Part model, mm, in its own coordinate system. A direction names the side the tool comes from. Coordinates: 2 decimals unless noted, no trailing zeros. Loops run counter-clockwise (first coordinate to the right, second up) from the corner with the lowest first, then second, coordinate; pieces in that order, holes last. Notation, with made-up numbers: M -10,58 L 34,58 A26 cw 34,89 Z; hole C 55.25,83 d3. An arc over 180 degrees is marked long. Use a Markdown table: item, result. Add a question column.
1) Band-saw the part on A-A (x = -15.5). List the corners of the cut face in (y, z), plus the area to 3 significant figures.
2) Pull direction Z, two halves, no side cores. Call faces 1 (the flat face through (-10, 1, -1)), 2 (the flat face through (-10, 1, -22)), 3 (the flat face through (-10, 2.5, -11)): released by +Z, released by -Z, zero draft, split by the parting line, or undercut.
3) Tool access for faces 4 (the flat face through (-20, 0.7, -0.5)), 5 (the flat face through (-10, 1, -21)), 6 (the flat face through (0, 0.7, -21.5)): list every direction of +Z, -Z, +X, -X, +Y, -Y with a clear straight run to the whole face (end or side of a thin tool).
4) Wall check: probe 1 along Z at (x, y) = (-13.5, 1.3); probe 2 along Y at (x, z) = (-15.5, -18). Give the ranges that are in metal, low to high. Write a range as from..to.
5) Band-saw the part on B-B (z = -14.75). List the corners of the cut face in (x, y), plus the area to 3 significant figures.
Autodesk Inventor part; units mm, degrees
ref_plane "YZ Plane" through (0, 0, 0) normal (1, 0, 0) x (0, 1, 0)
ref_plane "XZ Plane" through (0, 0, 0) normal (0, 1, 0) x (-1, 0, 0)
ref_plane "XY Plane" through (0, 0, 0) normal (0, 0, 1) x (1, 0, 0)
sketch "Skizze1" plane through (0, 0, 0) normal (0, 1, 0) x (-1, 0, 0)
  point P0 (0, 0)
sketch "Skizze2" plane through (0, 0, 0) normal (0, 1, 0) x (-1, 0, 0)
  line L0 (0, 0) -> (20, 0)
  line L1 (20, 0) -> (20, -22)
  line L2 (20, -22) -> (0, -22)
  line L3 (0, -22) -> (0, 0)
  line L4 (0, 0) -> (20, 0)
  line L5 (20, 0) -> (20, -1)
  line L6 (20, -1) -> (0, -1)
  line L7 (0, -1) -> (0, 0)
  line L8 (0, -22) -> (20, -22)
  line L9 (20, -22) -> (20, -21)
  line L10 (20, -21) -> (0, -21)
  line L11 (0, -21) -> (0, -22)
  dimension "d0" = 20
  dimension "d1" = 22
  dimension "d2" = 20
  dimension "d3" = 1
  dimension "d4" = 20
  dimension "d5" = 1
extrude "Extrusion1" add sketch "Skizze2" along normal blind 1.5 contours L0 L1 L6 L3 | L10 L1 L2 L3
sketch "Skizze3" plane through (0, 1.5, 0) normal (0, 1, 0) x (1, 0, 0)
  line L0 (1.5, 0) -> (-21.5, 0)
  line L1 (-21.5, 0) -> (-21.5, 22)
  line L2 (-21.5, 22) -> (1.5, 22)
  line L3 (1.5, 22) -> (1.5, 0)
  line L4 (-20, 22) -> (-20, 21)
  point P0 (0, 0)
  point P1 (-20, 21.5)
  dimension "d8" = 23
  dimension "d9" = 22
  dimension "d10" = 1.5
extrude "Extrusion2" add sketch "Skizze3" along normal blind 1
equation "\"Biegeradius\" = Stärke"
equation "\"BreiteBiegungsfreistellung\" = Stärke"
equation "\"TiefeBiegungsfreistellung\" = 0.5 * Stärke"
equation "\"GrößeEckenfreistellung\" = 4 * Stärke"
equation "\"MinimalRest\" = 2 * Stärke"
equation "\"Übergangsradius\" = Biegeradius"
equation "\"JacobiRadiusGröße\" = Biegeradius"
equation "\"Abstandsgröße\" = Stärke"
properties part number "V3_O3"
Entries:
| question | item | result |
|---|---|---|
| 1 | outline | M 0,-22 L 2.5,-22 L 2.5,0 L 0,0 L 0,-1 L 1.5,-1 L 1.5,-21 L 0,-21 Z |
| 1 | area | 25.0 mm2 |
| 2 | face 1 | undercut |
| 2 | face 2 | released by -Z |
| 2 | face 3 | zero draft |
| 3 | face 4 | +Z, -Z, -X, -Y |
| 3 | face 5 | +X, -X, -Y |
| 3 | face 6 | +Z, -Z, +X, -Y |
| 4 | probe 1 | -22..-21, -1..0 |
| 4 | probe 2 | 1.5..2.5 |
| 5 | outline | M -21.5,1.5 L 1.5,1.5 L 1.5,2.5 L -21.5,2.5 Z |
| 5 | area | 23.0 mm2 |
